Geometry: see drawing. Coordinates: mm, zero at the bounding-box minimum. Give positions to 0.01 mm unless a question says otherwise; leave off trailing zeros. Order: outer loops, then holes, each group sorted by start corner. A loop starts at its lowest first (then second) coordinate and runs counter-clockwise, first axis right, second up. Notation, with made-up numbers: M 51,69 L 107,69 A18 ccw 107,89 Z; hole C 31,79.5 d2. An arc over 180 degrees is marked long. Use a Markdown table: item, result.
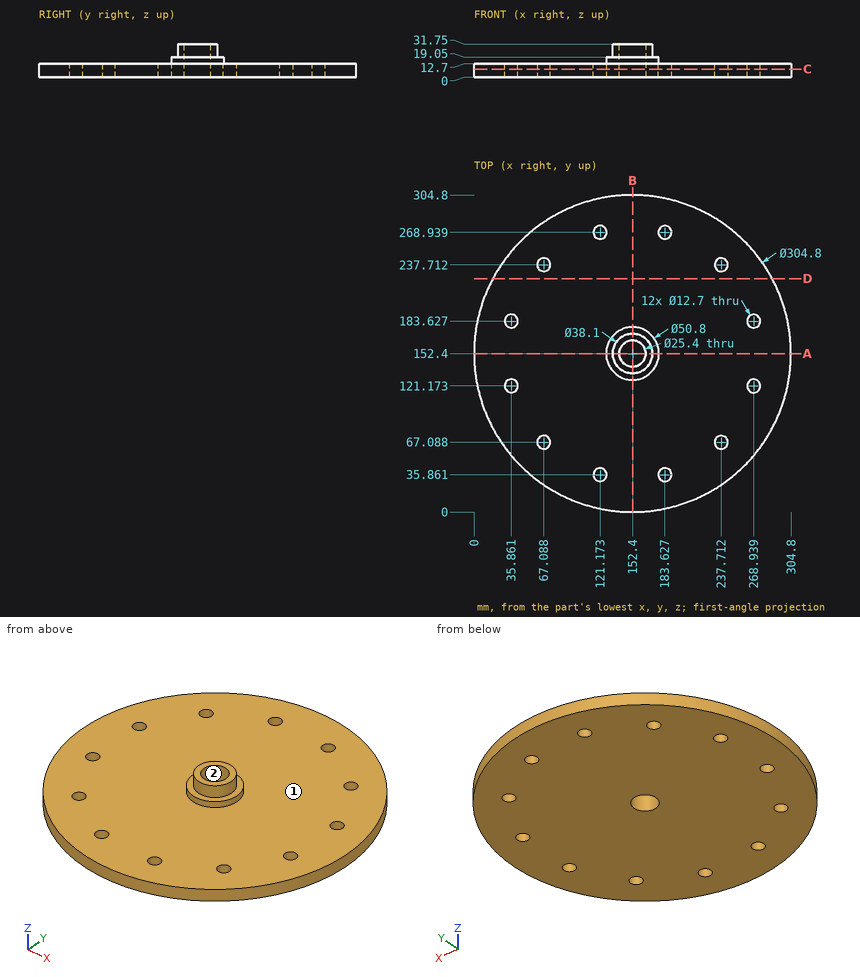
1) Cut plane D-D on y = 224.5. Return loops of the section in (x, z) (1 decimal).
Response values:
| item | result |
|---|---|
| outline | M 18.1,0 L 286.7,0 L 286.7,12.7 L 18.1,12.7 Z |
2) Cut plane A-A on y = 152.4. Return loops of the section in (x, z), and give its area (3 significant figures).
Response values:
| item | result |
|---|---|
| outline | M 0,0 L 139.7,0 L 139.7,31.75 L 133.35,31.75 L 133.35,19.05 L 127,19.05 L 127,12.7 L 0,12.7 Z; M 165.1,0 L 304.8,0 L 304.8,12.7 L 177.8,12.7 L 177.8,19.05 L 171.45,19.05 L 171.45,31.75 L 165.1,31.75 Z |
| area | 3,870 mm² |
3) Mould query, pull axis Y, two halves, no side actions, for the marked faces 1 and 2. Classes: released by +Y, released by -Y, zero draft, split by the parting line, or undercut.
Response values:
| item | result |
|---|---|
| face 1 | zero draft |
| face 2 | undercut |
4) Cut plane C-C on z = 7.5. State how many separate pieces and enclosed holes the cut face has, and give its area (3 significant figures).
Response values:
| item | result |
|---|---|
| separate pieces | 1 |
| enclosed holes | 13 |
| area | 70,900 mm² |
5) First-contact query: pin 1 Ø10 at (x, y) = (121.17, 268.94) entering from +Z; pin 2 Ø16.5 at (x, y) = (35.86, 121.17) entering from +Z; pin 3 Ø4 at (x, z) = (172.5, 14) entering from -Y; pin 4 Ø10 at (y, z) = (216, 6) entering from -X. Flat tips, straight axial feed; report the tip coordinate or a pass-through.
Response values:
| item | result |
|---|---|
| pin 1 | passes through |
| pin 2 | stops at z = 12.7 |
| pin 3 | stops at y = 1.14 |
| pin 4 | stops at x = 11.72 |
6) Material intervals for line 1 (Y direction, x = 121.5, z = 5.5) (1 decimal); line 2 (Z direction, x = 97.5, y = 110); line 3 (X direction, y = 264, z = 11) (1 decimal), sorted ascending. Write a range as from..to.
Response values:
| item | result |
|---|---|
| line 1 | y = 3.2..29.5, 42.2..262.6, 275.3..301.6 |
| line 2 | z = 0..12.7 |
| line 3 | x = 48.6..117.2, 125.2..179.6, 187.6..256.2 |
